Part model, mm, in its own coordinate system. Coordinates: 2 decimals unless noted, no trailing zeros. Loops run counter-clockwise (first coordinate to the right, second up) from the corner with the lowest first, then second, coordinate; pieces in that order, holes last. Notation, with made-up numbers: (-36, -17) -> (-19, -17) arc R21 ccw to (-19, 22) -> close; hole circle Ø7 at (57.25, 49.25). An arc over 180 degrees is marked (long way). One line per item, written item: value. Start each with the question number.
from build123d import *

# Parameters (mm, degrees)
F1_DEPTH = 360
F3_D     = 40
F5_D     = 5


with BuildPart() as f1:
    # F0 (on Top) → F1 (new body)
    with BuildSketch(Plane.XY):
        with BuildLine():
            Line((-14.4956890143, -14.4956890143), (0, 0))
            Line((0, 0), (-14.4956890143, 14.4956890143))
            ThreePointArc((-14.4956890143, 14.4956890143), (-16.2593773691, 13.3556947851), (-18.3356322814, 13.0404980289))
            ThreePointArc((-18.3356322814, 13.0404980289), (-21.4336385815, 6.8446429532), (-22.5, 4.93e-08))
            ThreePointArc((-22.5, 4.93e-08), (-21.4336385965, -6.8446429062), (-18.3356322814, -13.0404980289))
            ThreePointArc((-18.3356322814, -13.0404980289), (-16.2593773691, -13.3556947851), (-14.4956890143, -14.4956890143))
        make_face()
        with BuildLine():
            Line((-14.4956890143, 14.4956890143), (0, 0))
            Line((0, 0), (14.4956890143, 14.4956890143))
            ThreePointArc((14.4956890143, 14.4956890143), (13.3556947851, 16.2593773691), (13.0404980289, 18.3356322814))
            ThreePointArc((13.0404980289, 18.3356322814), (6.8446429123, 21.4336385946), (-3.64e-08, 22.5))
            ThreePointArc((-3.64e-08, 22.5), (-6.844642947, 21.4336385835), (-13.0404980289, 18.3356322814))
            ThreePointArc((-13.0404980289, 18.3356322814), (-13.0335422353, 18.1834982357), (-13.0312229203, 18.0312229203))
            ThreePointArc((-13.0312229203, 18.0312229203), (-13.4118252577, 16.1178057584), (-14.4956890143, 14.4956890143))
        make_face()
        with BuildLine():
            Line((0, 0), (22.5, 0))
            ThreePointArc((22.5, 0), (21.433638589, 6.8446429297), (18.3356322814, 13.0404980289))
            ThreePointArc((18.3356322814, 13.0404980289), (16.2593773691, 13.3556947851), (14.4956890143, 14.4956890143))
            Line((14.4956890143, 14.4956890143), (0, 0))
        make_face()
        with BuildLine():
            ThreePointArc((18.3356322814, -13.0404980289), (21.433638589, -6.8446429297), (22.5, 0))
            Line((22.5, 0), (0, 0))
            Line((0, 0), (14.4956890143, -14.4956890143))
            ThreePointArc((14.4956890143, -14.4956890143), (16.2593773691, -13.3556947851), (18.3356322814, -13.0404980289))
        make_face()
        with BuildLine():
            Line((14.4956890143, -14.4956890143), (0, 0))
            Line((0, 0), (-14.4956890143, -14.4956890143))
            ThreePointArc((-14.4956890143, -14.4956890143), (-13.4118252577, -16.1178057584), (-13.0312229203, -18.0312229203))
            ThreePointArc((-13.0312229203, -18.0312229203), (-13.0335422353, -18.1834982357), (-13.0404980289, -18.3356322814))
            ThreePointArc((-13.0404980289, -18.3356322814), (-6.8446429175, -21.4336385929), (2.56e-08, -22.5))
            ThreePointArc((2.56e-08, -22.5), (6.8446429419, -21.4336385851), (13.0404980289, -18.3356322814))
            ThreePointArc((13.0404980289, -18.3356322814), (13.3556947851, -16.2593773691), (14.4956890143, -14.4956890143))
        make_face()
        with BuildLine():
            ThreePointArc((-18.3356322814, 13.0404980289), (-16.2593773691, 13.3556947851), (-14.4956890143, 14.4956890143))
            Line((-14.4956890143, 14.4956890143), (-15.9099025767, 15.9099025767))
            ThreePointArc((-15.9099025767, 15.9099025767), (-17.18276855, 14.5259238934), (-18.3356322814, 13.0404980289))
        make_face()
        with BuildLine():
            Line((-15.9099025767, 15.9099025767), (-14.4956890143, 14.4956890143))
            ThreePointArc((-14.4956890143, 14.4956890143), (-13.4118252577, 16.1178057584), (-13.0312229203, 18.0312229203))
            ThreePointArc((-13.0312229203, 18.0312229203), (-13.0335422353, 18.1834982357), (-13.0404980289, 18.3356322814))
            ThreePointArc((-13.0404980289, 18.3356322814), (-14.5259238934, 17.18276855), (-15.9099025767, 15.9099025767))
        make_face()
        with BuildLine():
            Line((-18.0312229203, 18.0312229203), (-15.9099025767, 15.9099025767))
            ThreePointArc((-15.9099025767, 15.9099025767), (-14.5259238934, 17.18276855), (-13.0404980289, 18.3356322814))
            ThreePointArc((-13.0404980289, 18.3356322814), (-13.8579312806, 20.7850633096), (-15.7884497682, 22.5))
            Line((-15.7884497682, 22.5), (-20.2739960723, 22.5))
            ThreePointArc((-20.2739960723, 22.5), (-20.9578154473, 22.0852402094), (-21.5667568262, 21.5667568262))
            Line((-21.5667568262, 21.5667568262), (-18.0312229203, 18.0312229203))
        make_face()
        with BuildLine():
            ThreePointArc((-18.3356322814, 13.0404980289), (-17.18276855, 14.5259238934), (-15.9099025767, 15.9099025767))
            Line((-15.9099025767, 15.9099025767), (-18.0312229203, 18.0312229203))
            Line((-18.0312229203, 18.0312229203), (-21.5667568262, 21.5667568262))
            ThreePointArc((-21.5667568262, 21.5667568262), (-22.0852402094, 20.9578154473), (-22.5, 20.2739960723))
            Line((-22.5, 20.2739960723), (-22.5, 15.7884497682))
            ThreePointArc((-22.5, 15.7884497682), (-20.7850633096, 13.8579312806), (-18.3356322814, 13.0404980289))
        make_face()
        with BuildLine():
            ThreePointArc((13.0404980289, 18.3356322814), (14.5259238934, 17.18276855), (15.9099025767, 15.9099025767))
            Line((15.9099025767, 15.9099025767), (21.5667568262, 21.5667568262))
            ThreePointArc((21.5667568262, 21.5667568262), (20.9578154473, 22.0852402094), (20.2739960723, 22.5))
            Line((20.2739960723, 22.5), (15.7884497682, 22.5))
            ThreePointArc((15.7884497682, 22.5), (13.8579312806, 20.7850633096), (13.0404980289, 18.3356322814))
        make_face()
        with BuildLine():
            ThreePointArc((15.9099025767, 15.9099025767), (17.18276855, 14.5259238934), (18.3356322814, 13.0404980289))
            ThreePointArc((18.3356322814, 13.0404980289), (20.7850633096, 13.8579312806), (22.5, 15.7884497682))
            Line((22.5, 15.7884497682), (22.5, 20.2739960723))
            ThreePointArc((22.5, 20.2739960723), (22.0852402094, 20.9578154473), (21.5667568262, 21.5667568262))
            Line((21.5667568262, 21.5667568262), (15.9099025767, 15.9099025767))
        make_face()
        with BuildLine():
            ThreePointArc((14.4956890143, 14.4956890143), (16.2593773691, 13.3556947851), (18.3356322814, 13.0404980289))
            ThreePointArc((18.3356322814, 13.0404980289), (17.18276855, 14.5259238934), (15.9099025767, 15.9099025767))
            Line((15.9099025767, 15.9099025767), (14.4956890143, 14.4956890143))
        make_face()
        with BuildLine():
            Line((14.4956890143, 14.4956890143), (15.9099025767, 15.9099025767))
            ThreePointArc((15.9099025767, 15.9099025767), (14.5259238934, 17.18276855), (13.0404980289, 18.3356322814))
            ThreePointArc((13.0404980289, 18.3356322814), (13.3556947851, 16.2593773691), (14.4956890143, 14.4956890143))
        make_face()
        with BuildLine():
            Line((21.5667568262, -21.5667568262), (15.9099025767, -15.9099025767))
            ThreePointArc((15.9099025767, -15.9099025767), (14.5259238934, -17.18276855), (13.0404980289, -18.3356322814))
            ThreePointArc((13.0404980289, -18.3356322814), (13.8579312806, -20.7850633096), (15.7884497682, -22.5))
            Line((15.7884497682, -22.5), (20.2739960723, -22.5))
            ThreePointArc((20.2739960723, -22.5), (20.9578154473, -22.0852402094), (21.5667568262, -21.5667568262))
        make_face()
        with BuildLine():
            ThreePointArc((22.5, -15.7884497682), (20.7850633096, -13.8579312806), (18.3356322814, -13.0404980289))
            ThreePointArc((18.3356322814, -13.0404980289), (17.18276855, -14.5259238934), (15.9099025767, -15.9099025767))
            Line((15.9099025767, -15.9099025767), (21.5667568262, -21.5667568262))
            ThreePointArc((21.5667568262, -21.5667568262), (22.0852402094, -20.9578154473), (22.5, -20.2739960723))
            Line((22.5, -20.2739960723), (22.5, -15.7884497682))
        make_face()
        with BuildLine():
            ThreePointArc((15.9099025767, -15.9099025767), (17.18276855, -14.5259238934), (18.3356322814, -13.0404980289))
            ThreePointArc((18.3356322814, -13.0404980289), (16.2593773691, -13.3556947851), (14.4956890143, -14.4956890143))
            Line((14.4956890143, -14.4956890143), (15.9099025767, -15.9099025767))
        make_face()
        with BuildLine():
            ThreePointArc((13.0404980289, -18.3356322814), (14.5259238934, -17.18276855), (15.9099025767, -15.9099025767))
            Line((15.9099025767, -15.9099025767), (14.4956890143, -14.4956890143))
            ThreePointArc((14.4956890143, -14.4956890143), (13.3556947851, -16.2593773691), (13.0404980289, -18.3356322814))
        make_face()
        with BuildLine():
            Line((-21.5667568262, -21.5667568262), (-15.9099025767, -15.9099025767))
            ThreePointArc((-15.9099025767, -15.9099025767), (-17.18276855, -14.5259238934), (-18.3356322814, -13.0404980289))
            ThreePointArc((-18.3356322814, -13.0404980289), (-20.7850633096, -13.8579312806), (-22.5, -15.7884497682))
            Line((-22.5, -15.7884497682), (-22.5, -20.2739960723))
            ThreePointArc((-22.5, -20.2739960723), (-22.0852402094, -20.9578154473), (-21.5667568262, -21.5667568262))
        make_face()
        with BuildLine():
            ThreePointArc((-13.0404980289, -18.3356322814), (-14.5259238934, -17.18276855), (-15.9099025767, -15.9099025767))
            Line((-15.9099025767, -15.9099025767), (-21.5667568262, -21.5667568262))
            ThreePointArc((-21.5667568262, -21.5667568262), (-20.9578154473, -22.0852402094), (-20.2739960723, -22.5))
            Line((-20.2739960723, -22.5), (-15.7884497682, -22.5))
            ThreePointArc((-15.7884497682, -22.5), (-13.8579312806, -20.7850633096), (-13.0404980289, -18.3356322814))
        make_face()
        with BuildLine():
            ThreePointArc((-13.0312229203, -18.0312229203), (-13.4118252577, -16.1178057584), (-14.4956890143, -14.4956890143))
            Line((-14.4956890143, -14.4956890143), (-15.9099025767, -15.9099025767))
            ThreePointArc((-15.9099025767, -15.9099025767), (-14.5259238934, -17.18276855), (-13.0404980289, -18.3356322814))
            ThreePointArc((-13.0404980289, -18.3356322814), (-13.0335422353, -18.1834982357), (-13.0312229203, -18.0312229203))
        make_face()
        with BuildLine():
            Line((-15.9099025767, -15.9099025767), (-14.4956890143, -14.4956890143))
            ThreePointArc((-14.4956890143, -14.4956890143), (-16.2593773691, -13.3556947851), (-18.3356322814, -13.0404980289))
            ThreePointArc((-18.3356322814, -13.0404980289), (-17.18276855, -14.5259238934), (-15.9099025767, -15.9099025767))
        make_face()
    extrude(amount=F1_DEPTH)

    # F3 (through all)
    with Locations(Plane.XY.offset(360)):
        with Locations((0, 0)):
            Hole(F3_D / 2)

    # F5 (through all)
    with Locations(Plane.XY.offset(360)):
        with Locations((-18.0312229203, 18.0312229203), (18.0312229203, 18.0312229203), (18.0312229203, -18.0312229203), (-18.0312229203, -18.0312229203)):
            Hole(F5_D / 2)


solid = f1.part
1) Slice it at B-B (x = -6). Give the cut face in (y, z).
2) Probe line 1 (Y direction, x = -1.5, z = 15.5); line 2 (Y direction, x = 16.5, z = 108); line 3 (X direction, y = 17.5, z = 200.5). List the from-to ranges inside material, lowest first. Write a range as from..to.
3) Pull direction Y, two halves, no side cores. Call faces 1 (the flat face through (-18.4, 8.4, 0)), 2 (the cylindrical face through (4.336, -19.524, 177.48)): +Y half, -Y half, draft (parallel to the pull), parting line (faces both ways), or undercut.
4) Pin check, flat tips, straight feed: pin 1 Ø3 at (x, z) = (-14.5, 313) entering from -Y; pin 2 Ø5 at (x, z) = (8, 311) entering from -Y; pin 3 Ø10 at (x, z) = (9.5, 66) entering from -Y; pin 4 Ø8 at (x, z) = (8, 209.5) entering from +Y. Stop position of each tip, or through.
5) Slice it at A-A (y = -9.5). Give the cut face in (x, z), then the cut area to 3 significant figures.
6) Slice it at C-C (z = 197). State how many separate pieces and enclosed holes the cut face has, then the cut area to 3 significant figures.
Check sheet entries:
1. outline: (-21.69, 0) -> (-19.08, 0) -> (-19.08, 360) -> (-21.69, 360) -> close; (19.08, 0) -> (21.69, 0) -> (21.69, 360) -> (19.08, 360) -> close
2. line 1: y = -22.45..-19.94, 19.94..22.45
2. line 2: y = -22.5..-20.01, -16.06..-11.3, 11.3..16.06, 20.01..22.5
2. line 3: x = -22.5..-20.47, -15.59..-9.68, 9.68..15.59, 20.47..22.5
3. face 1: draft
3. face 2: undercut
4. pin 1: stops at y = -22.5
4. pin 2: stops at y = -21.82
4. pin 3: stops at y = -22.05
4. pin 4: stops at y = 22.14
5. outline: (-20.4, 0) -> (-17.6, 0) -> (-17.6, 360) -> (-20.4, 360) -> close; (17.6, 0) -> (20.4, 0) -> (20.4, 360) -> (17.6, 360) -> close
5. area: 2,010 mm^2
6. separate pieces: 1
6. enclosed holes: 5
6. area: 515 mm^2
